Model file for the job. Use its own axes, mm. A direction names the side the tool comes from. Give positions to 0.01 mm unless a question says otherwise; leave off trailing zeros. Order: outer loops, then holes, each group sorted by start corner. A loop starts at its lowest first (then second) coordinate and runs counter-clockwise, first axis right, second up. Notation, with made-up numbers: M 64.5,-20.5 L 103.5,-20.5 A30 cw 103.5,8.5 Z; hole C 36.5,78.25 d1. An arc over 180 degrees is marked long. Return JSON: item names as keys, results as strings. Group by question number.
1. 3-axis set-ups, long thin cutter, end or side, ignore diameter. For faces 4 (the face through (-2.83, 3.087, 187.325)), 5 (the face through (2.83, 3.087, -187.325)), 6 (the face through (0, -5, -200)): which of +Z, -Z, +X, -X, +Y, -Y reach the whole face in a straight line?
2. Slice it at A-A on z = 63. List the corners of the cut face in (x, y).
3. Pin check, flat tips, straight feed: pin 1 (1.5 mm diameter, centred on x = 8, z = 131, fed in from +Y); pin 2 (6 mm diameter, centred on y = -5.5, z = -128.5, fed in from -X); pin 3 (6 mm diameter, centred on x = -4.5, z = -121, fed in from -Y). Stop position of each tip, or through.
4. Two-plate mould, pull along Y, no slides. Class faces 1 (the face through (0, -5, 200)), 2 (the face through (0.71, 0.16, -172.92)), 3 (the face through (11.923, 3.755, 2.8)): released by +Y, released by -Y, zero draft, split by the parting line, or undercut.
5. Slice it at B-B on y = -9. List the corners of the cut face in (x, z).
6. Wall check: probe 1 along Y at (x, z) = (0, 194.75); probe 2 along Y at (x, z) = (-1.25, 181); probe 3 along X at (y, z) = (-3.5, 170.5). Give the ranges that are in metal, low to high. Write a range as [from, to].
Autodesk Inventor part; units mm, degrees
ref_plane "YZ Plane" through (0, 0, 0) normal (1, 0, 0) x (0, 1, 0)
ref_plane "XZ Plane" through (0, 0, 0) normal (0, 1, 0) x (-1, 0, 0)
ref_plane "XY Plane" through (0, 0, 0) normal (0, 0, 1) x (1, 0, 0)
sketch "Sketch1" plane through (0, 0, 0) normal (0, 0, 1) x (1, 0, 0)
  circle A0 centre (0, 0) radius 12.5
  dimension "d0" = 25
extrude "Extrusion1" add sketch "Sketch1" along normal mid plane 400
sketch "Sketch2" plane through (0, 0, 200) normal (0, 0, 1) x (1, 0, 0)
  circle A0 centre (0, 0) radius 12.5
hole "Hole1" at (0, 0, 200) direction (0, 0, -1) diameter 8.376 depth 25 tip angle 118
mirror "Mirror1" about plane through (0, 0, 0) normal (0, 0, 1) of "Hole1"
properties part number "ADSK-MH-10018" material "Steel, Mild"
Result:
{
 "1": {"face 4": "+Z", "face 5": "-Z", "face 6": "-Z, +X, -X, +Y, -Y"},
 "2": {"outline": "C 0,0 d25"},
 "3": {"pin 1": "stops at y = 10.18", "pin 2": "stops at x = -12.25", "pin 3": "stops at y = -12.41"},
 "4": {"face 1": "zero draft", "face 2": "undercut", "face 3": "split by the parting line"},
 "5": {"outline": "M -8.67,-200 L 8.67,-200 L 8.67,200 L -8.67,200 Z"},
 "6": {"probe 1": "y = [-12.5, -4.19], [4.19, 12.5]", "probe 2": "y = [-12.44, -4], [4, 12.44]", "probe 3": "x = [-12, 12]"}
}
